from build123d import *

# Parameters (mm, degrees)
SKETCH_1_W          = 20
SKETCH_1_H          = 20
SKETCH_1_W_2        = 17
SKETCH_1_H_2        = 17
EXTRUDE_1_DEPTH     = 206
SKETCH_2_R          = 1.575
CUT_EXTRUDE_1_DEPTH = 208.932681414
SKETCH_3_R          = 1.6
CUT_EXTRUDE_2_DEPTH = 208.932681414


with BuildPart() as part:
    # 草图1 → 拉伸-薄壁1 (new body)
    with BuildSketch(Plane.XY):
        with Locations((10, -10)):
            Rectangle(SKETCH_1_W, SKETCH_1_H)
        with Locations((10, -10)):
            Rectangle(SKETCH_1_W_2, SKETCH_1_H_2, mode=Mode.SUBTRACT)
    extrude(amount=EXTRUDE_1_DEPTH)

    # 草图2 → 切除-拉伸1 (cut, through all)
    with BuildSketch(Plane(origin=(0, 0, 0), x_dir=(1, 0, 0), z_dir=(0, 1, 0))):
        with Locations(Location((5, -191, 0), (0, 0, 270))):
            Circle(SKETCH_2_R)
        with Locations(Location((15, -191, 0), (0, 0, 90))):
            Circle(SKETCH_2_R)
        with Locations(Location((15, -201, 0), (0, 0, 270))):
            Circle(SKETCH_2_R)
        with Locations(Location((5, -201, 0), (0, 0, 90))):
            Circle(SKETCH_2_R)
        with Locations(Location((5, -25, 0), (0, 0, 270))):
            Circle(SKETCH_2_R)
        with Locations(Location((15, -25, 0), (0, 0, 90))):
            Circle(SKETCH_2_R)
        with Locations(Location((15, -35, 0), (0, 0, 270))):
            Circle(SKETCH_2_R)
        with Locations(Location((5, -35, 0), (0, 0, 90))):
            Circle(SKETCH_2_R)
        with Locations(Location((5, -75, 0), (0, 0, 270))):
            Circle(SKETCH_2_R)
        with Locations(Location((15, -75, 0), (0, 0, 90))):
            Circle(SKETCH_2_R)
        with Locations(Location((15, -85, 0), (0, 0, 270))):
            Circle(SKETCH_2_R)
        with Locations(Location((5, -85, 0), (0, 0, 90))):
            Circle(SKETCH_2_R)
    extrude(amount=-CUT_EXTRUDE_1_DEPTH, mode=Mode.SUBTRACT)

    # 草图3 → 切除-拉伸2 (cut, through all)
    with BuildSketch(Plane.ZY):
        with Locations(Location((118, -5, 0), (0, 0, 270))):
            Circle(SKETCH_3_R)
        with Locations((128, -5)):
            Circle(SKETCH_3_R)
        with Locations(Location((128, -15, 0), (0, 0, 270))):
            Circle(SKETCH_3_R)
        with Locations((118, -15)):
            Circle(SKETCH_3_R)
        with Locations(Location((168, -15, 0), (0, 0, 270))):
            Circle(SKETCH_3_R)
        with Locations((158, -15)):
            Circle(SKETCH_3_R)
        with Locations(Location((158, -5, 0), (0, 0, 270))):
            Circle(SKETCH_3_R)
        with Locations((168, -5)):
            Circle(SKETCH_3_R)
        with Locations(Location((30, -5, 0), (0, 0, 270))):
            Circle(SKETCH_3_R)
        with Locations((40, -5)):
            Circle(SKETCH_3_R)
        with Locations(Location((40, -15, 0), (0, 0, 270))):
            Circle(SKETCH_3_R)
        with Locations((30, -15)):
            Circle(SKETCH_3_R)
        with Locations(Location((80, -10, 0), (0, 0, 270))):
            Circle(SKETCH_3_R)
        with Locations(Location((77.307692308, -3.538461538, 0), (0, 0, 270))):
            Circle(SKETCH_3_R)
    extrude(amount=-CUT_EXTRUDE_2_DEPTH, mode=Mode.SUBTRACT)


solid = part.part
CAD build for the part. Positions are in the model's coordinates, mm. A direction names the side the tool comes from. Coordinates: 2 decimals unless noted, no trailing zeros. Loops run counter-clockwise (first coordinate to the right, second up) from the corner with the lowest first, then second, coordinate; pieces in that order, holes last. Notation, with made-up numbers: (9.5, 56.25) -> (43.5, 56.25) arc R32 ccw to (43.5, 90.25) -> close; hole circle Ø9 at (40.25, -5). An arc over 180 degrees is marked (long way). One line per item, written item: value.
1. Drill centre lines: line 1 (X direction, y = -19.55, z = 191) (3 decimals); line 2 (X direction, y = -14, z = 196); line 3 (Y direction, x = 9.5, z = 166.5). Where is each one in solid material? Low to high. Write a range as [from, to].
Answers:
line 1: x = [0, 3.425], [6.575, 13.425], [16.575, 20]
line 2: x = [0, 1.5], [18.5, 20]
line 3: y = [-20, -18.5], [-1.5, 0]
2. Which spindle directions (+Z, -Z, +X, -X, +Y, -Y) get a long thin tool onto all of the face, cutting with end or side? Do faces 1 (the face through (10, -18.5, 102)), 2 (the face through (0.74, -5.61, 129.48)). Say none if no direction does.
Answers:
face 1: +Z, -Z
face 2: +X, -X
3. Slice it at A-A on z = 19.5. Write the cut outline in (x, y).
Answers:
outline: (0, -20) -> (20, -20) -> (20, 0) -> (0, 0) -> close; hole (1.5, -18.5) -> (18.5, -18.5) -> (18.5, -1.5) -> (1.5, -1.5) -> close
4. Pull direction Y, two halves, no side cores. Call faces 3 (the face through (19.24, -5.61, 169.48)), 4 (the face through (14.527, -19.24, 189.498)), 5 (the face through (10, 0, 102)): pulls with the +Y half, pulls with the -Y half, needs draft (parallel to the pull), parting line crosses it, or undercut.
Answers:
face 3: undercut
face 4: needs draft
face 5: pulls with the +Y half
